```python
from build123d import *

# Parameters (mm, degrees)
SKETCH_1_W               = 35
SKETCH_1_H               = 60
EXTRUDE_1_DEPTH          = 2
HOLE_WIZARD_1_D          = 3.5
PATTERN_CIRCULAR_1_COUNT = 6
SKETCH_5_R               = 11.5
CUT_EXTRUDE_1_DEPTH      = 2
SKETCH_11_W              = 35
SKETCH_11_H              = 6
EXTRUDE_2_DEPTH          = 7
SKETCH_12_W              = 2.85
SKETCH_12_H              = 5
CUT_EXTRUDE_3_DEPTH      = 64.144675152
HOLE_WIZARD_2_D          = 3.5
HOLE_WIZARD_2_DEPTH      = 2


with BuildPart() as part:
    # 草图1 → 凸台-拉伸1 (new body)
    with BuildSketch(Plane(origin=(0, 0, 0), x_dir=(1, 0, 0), z_dir=(0, 1, 0))):
        Rectangle(SKETCH_1_W, SKETCH_1_H)
    extrude(amount=EXTRUDE_1_DEPTH)

    # 孔1 (through all)
    with Locations(Plane(origin=(0, 2, 0), x_dir=(1, 0, 0), z_dir=(0, 1, 0))):
        with Locations((0, 14)):
            hole_wizard_1 = Hole(HOLE_WIZARD_1_D / 2)

    # 阵列(圆周)1: 孔1 ×6 about axis
    pattern_circular_1_axis = Axis((0, 0, 0), (0, 1, 0))
    for i in range(1, PATTERN_CIRCULAR_1_COUNT):
        add(hole_wizard_1.rotate(pattern_circular_1_axis, i * 360 / PATTERN_CIRCULAR_1_COUNT), mode=Mode.SUBTRACT)

    # 草图5 → 切除-拉伸1 (cut)
    with BuildSketch(Plane(origin=(0, 2, 0), x_dir=(1, 0, 0), z_dir=(0, 1, 0))):
        with Locations(Location((0, 0, 0), (0, 0, 270))):
            Circle(SKETCH_5_R)
    extrude(amount=-CUT_EXTRUDE_1_DEPTH, mode=Mode.SUBTRACT)

    # 草图11 → 凸台-拉伸2 (add)
    with BuildSketch(Plane(origin=(0, 2, 0), x_dir=(1, 0, 0), z_dir=(0, 1, 0))):
        with Locations((0, -27)):
            Rectangle(SKETCH_11_W, SKETCH_11_H)
        with Locations((0, 27)):
            Rectangle(SKETCH_11_W, SKETCH_11_H)
    extrude(amount=EXTRUDE_2_DEPTH)

    # 草图12 → 切除-拉伸3 (cut, through all)
    with BuildSketch(Plane.XY.offset(30)):
        with Locations((-10.175, 4.5)):
            Rectangle(SKETCH_12_W, SKETCH_12_H)
        with Locations((-7.325, 4.5)):
            Rectangle(SKETCH_12_W, SKETCH_12_H)
        with Locations((10.175, 4.5)):
            Rectangle(SKETCH_12_W, SKETCH_12_H)
        with Locations((7.325, 4.5)):
            Rectangle(SKETCH_12_W, SKETCH_12_H)
    extrude(amount=-CUT_EXTRUDE_3_DEPTH, mode=Mode.SUBTRACT)

    # 孔2
    with Locations(Plane(origin=(0, 9, 0), x_dir=(1, 0, 0), z_dir=(0, 1, 0))):
        with Locations((-8.75, 27), (8.75, 27), (-8.75, -27), (8.75, -27)):
            Hole(HOLE_WIZARD_2_D / 2, depth=HOLE_WIZARD_2_DEPTH)


solid = part.part
```
Input: part model. Units: mm. Frame: model coordinates. A direction names the side the tool comes from. Give positions to 0.01 mm unless a question says otherwise; leave off trailing zeros. Order: outer loops, then holes, each group sorted by start corner. A loop starts at its lowest first (then second) coordinate and runs counter-clockwise, first axis right, second up. Notation, with made-up numbers: (-13, -30) -> (15, -30) arc R10 cw to (15, -16) -> close; hole circle Ø11 at (-5.5, 79.25). An arc over 180 degrees is marked (long way). Write each question's results on one line, items separated by ' | '. Start each with the question number.
Item 1: Set-up query: faces 1 (the flat face through (-5.9, 4, 27)), 2 (the cylindrical face through (0.228, 0.986, -15.735)), 3 (the cylindrical face through (8.978, 7.986, 25.265)). Return all of +Z, -Z, +X, -X, +Y, -Y with unobstructed straight access to the full face (end or side cutting, diameter ignored); none if empty.
Item 2: Cut plane B-B on y = 3. Return the cut outline in (x, z), then the cut area to 3 significant figures.
Item 3: Line query: line 1 (X direction, y = 8.45, z = -27); line 2 (Z direction, x = -8.75, y = 8.3); line 3 (Z direction, x = 0, y = 0.9). Output: solid intervals per line, ascending.
Item 4: Mould query, pull axis Z, two halves, no side actions, for faces 4 (the cylindrical face through (7.809, 7.986, -28.476)), 5 (the cylindrical face through (-9.691, 7.986, -28.476)), 6 (the flat face through (5.9, 4, 27)). Classes: pulls with the +Z half, pulls with the -Z half, needs draft (parallel to the pull), parting line crosses it, or undercut.
Item 5: Cut plane C-C on y = 7.75. Return the cut outline in (x, z), then the cut area to 3 significant figures.
Item 6: Contact query for a flat-ended pin moving along its axis: P1, Ø6, axis at x = 8.5, z = -3.5, coming from the +Y side. Output: stop coordinate, or through.
Item 7: Cut plane A-A on z = -14. Return the cut outline in (x, y).
Item 8: Cut plane D-D on x = -9. Return the cut outline in (y, z).
Established:
1) face 1: +Z, -Z | face 2: +Y, -Y | face 3: +Y
2) outline: (-17.5, -30) -> (-11.6, -30) -> (-11.6, -24) -> (-17.5, -24) -> close; (-17.5, 24) -> (-11.6, 24) -> (-11.6, 30) -> (-17.5, 30) -> close; (-5.9, -30) -> (5.9, -30) -> (5.9, -24) -> (-5.9, -24) -> close; (-5.9, 24) -> (5.9, 24) -> (5.9, 30) -> (-5.9, 30) -> close; (11.6, -30) -> (17.5, -30) -> (17.5, -24) -> (11.6, -24) -> close; (11.6, 24) -> (17.5, 24) -> (17.5, 30) -> (11.6, 30) -> close | area: 283 mm^2
3) line 1: -17.5 to -10.5, -7 to 7, 10.5 to 17.5 | line 2: -30 to -28.75, -25.25 to -24, 24 to 25.25, 28.75 to 30 | line 3: -30 to -15.75, -12.25 to -11.5, 11.5 to 12.25, 15.75 to 30
4) face 4: undercut | face 5: undercut | face 6: needs draft
5) outline: (-17.5, -30) -> (17.5, -30) -> (17.5, -24) -> (-17.5, -24) -> close; (-17.5, 24) -> (17.5, 24) -> (17.5, 30) -> (-17.5, 30) -> close; hole circle Ø3.5 at (-8.75, -27); hole circle Ø3.5 at (-8.75, 27); hole circle Ø3.5 at (8.75, -27); hole circle Ø3.5 at (8.75, 27) | area: 382 mm^2
6) P1: y = 2
7) outline: (-17.5, 0) -> (-1.75, 0) -> (-1.75, 2) -> (-17.5, 2) -> close; (1.75, 0) -> (17.5, 0) -> (17.5, 2) -> (1.75, 2) -> close
8) outline: (0, -30) -> (2, -30) -> (2, -7.16) -> (0, -7.16) -> close; (0, 7.16) -> (2, 7.16) -> (2, 30) -> (0, 30) -> close; (7, -30) -> (9, -30) -> (9, -28.73) -> (7, -28.73) -> close; (7, -25.27) -> (9, -25.27) -> (9, -24) -> (7, -24) -> close; (7, 24) -> (9, 24) -> (9, 25.27) -> (7, 25.27) -> close; (7, 28.73) -> (9, 28.73) -> (9, 30) -> (7, 30) -> close
